Could you check a few things on this drawing? It's one solid part, dimensions in mm from its lowest x, y, z. A direction names the side the tool comes from. Give positions to 0.01 mm unless a question says otherwise; leave off trailing zeros. Order: outer loops, then holes, each group sorted by start corner. A loop starts at its lowest first (then second) coordinate and runs counter-clockwise, first axis right, second up. Notation, with made-up numbers: M -35.5,58 L -4.5,58 A22 cw -4.5,68 Z; hole C 89.5,-34.5 d9. An arc over 180 degrees is marked long. Return JSON: item names as keys, results as strings. Group by question number.
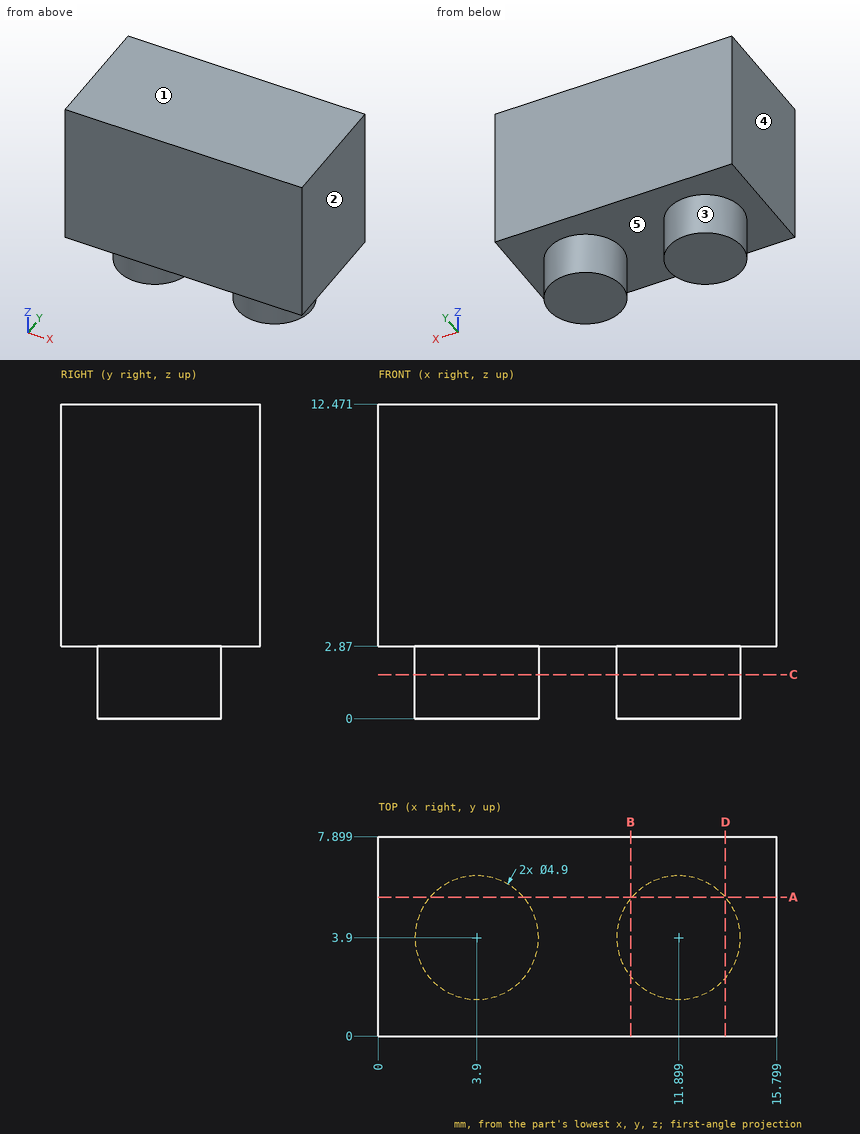
1. Imagine slicing it at B-B, the plane x = 10. Please give me the cut outline in (y, z).
2. Which directions (+Z, -Z, +X, -X, +Y, -Y) give clear straight access to the entire face, cutting with the end or side of a thin tool? Please do the marked faces 4 and 5.
3. Imagine slicing it at D-D, the plane x = 13.75. Please give me the cut outline in (y, z) (1 decimal).
4. I need wall thicknesses on L1, parallel to X at y = 4, z = 2.5; L2, parallel to Z at x = 10.25, y = 1.5; L3, parallel to Y at x = 4, z = 1.5. Which ranges of each line are inside material? Lowest first, please. Write a range as from..to.
5. If we mould it in two halves opening along X, with no side actions, what happens to the marked faces 1, 2 and 3? For each: pulls with the +X half, pulls with the -X half, needs draft (parallel to the pull), parting line crosses it, or undercut.
6. Imagine slicing it at A-A, the plane y = 5.5. Please give me the cut outline in (x, z) (1 decimal), plus the area to 3 significant figures.
7. Imagine slicing it at C-C, the plane z = 1.75. Please give me the cut outline in (x, y), plus the area to 3 significant figures.
Values:
{
 "1": {"outline": "M 0,2.87 L 2.35,2.87 L 2.35,0 L 5.45,0 L 5.45,2.87 L 7.9,2.87 L 7.9,12.47 L 0,12.47 Z"},
 "2": {"face 4": "+Z, -Z, -X, +Y, -Y", "face 5": "-Z"},
 "3": {"outline": "M 0,2.9 L 2.3,2.9 L 2.3,0 L 5.5,0 L 5.5,2.9 L 7.9,2.9 L 7.9,12.5 L 0,12.5 Z"},
 "4": {"L1": "x = 1.45..6.35, 9.45..14.35", "L2": "z = 2.87..12.47", "L3": "y = 1.45..6.35"},
 "5": {"face 1": "needs draft", "face 2": "pulls with the +X half", "face 3": "undercut"},
 "6": {"outline": "M 0,2.9 L 2,2.9 L 2,0 L 5.8,0 L 5.8,2.9 L 10,2.9 L 10,0 L 13.8,0 L 13.8,2.9 L 15.8,2.9 L 15.8,12.5 L 0,12.5 Z", "area": "173 mm²"},
 "7": {"outline": "C 3.9,3.9 d4.9; C 11.9,3.9 d4.9", "area": "37.7 mm²"}
}
